from build123d import *

# Parameters (mm, degrees)
SKETCH_3_R          = 2
CUT_EXTRUDE_1_DEPTH = 10


with BuildPart() as part:
    # 草图1 → 旋转3 (revolve)
    with BuildSketch(Plane.XY):
        with BuildLine():
            Line((-14.38749457, 17), (-12.38749457, 17))
            Line((-12.38749457, 17), (-12.38749457, 6.523034438))
            ThreePointArc((-12.38749457, 6.523034438), (-13.590896291, 3.359693142), (-14, 0))
            Line((-14, 0), (-16, 0))
            ThreePointArc((-16, 0), (-15.591663047, 3.591663047), (-14.38749457, 7))
            Line((-14.38749457, 7), (-14.38749457, 17))
        make_face()
    revolve(axis=Axis((-26.155193714, 0, 0), (1, 0, 0)))

    # 草图2 → 切除-旋转1 (revolve, cut)
    with BuildSketch(Plane.XY):
        Polygon((-10.99354471, 5.03904502), (-18.623280316, 7.444691416), (-19.074339015, 6.01411599), (-11.444603409, 3.608469594), align=None)
    cut_revolve_1 = revolve(axis=Axis((0, 0, 0), (-0.9537169507482267, 0.30070579950427373, 0)), mode=Mode.SUBTRACT)

    # 镜向1: 切除-旋转1 across plane
    add(cut_revolve_1.mirror(Plane.ZX), mode=Mode.SUBTRACT)

    # 草图3 → 切除-拉伸1 (cut)
    with BuildSketch(Plane.ZY.offset(14.38749457)):
        with Locations((0, 12)):
            Circle(SKETCH_3_R)
        with Locations((10.392304845, -6)):
            Circle(SKETCH_3_R)
        with Locations((-10.392304845, -6)):
            Circle(SKETCH_3_R)
    extrude(amount=-CUT_EXTRUDE_1_DEPTH, mode=Mode.SUBTRACT)


solid = part.part
Build history of the part. All positions in model axes, mm. Round coordinates to 2 decimals unless told otherwise and drop trailing zeros. Loops run counter-clockwise (first coordinate to the right, second up) from the corner with the lowest first, then second, coordinate; pieces in that order, holes last. Notation, with made-up numbers: (-6, 15.5) -> (43, 15.5) arc R16 ccw to (43, 23.5) -> close; hole circle Ø7 at (59, 5.25). An arc over 180 degrees is marked (long way). Use CSV: the item, a comma, the result in double quotes. Start each with the question number.
Q1. Saw through at C-C on z = 0. Give the cut face in (x, y), and give its area (3 significant figures).
Q2. Saw through at B-B on z = -10.5. Give the cut face in (x, y).
Q3. Flat gauge pins, fed straight in: pin 1 Ø2 at (x, z) = (-13, -11) entering from -Y; pin 2 Ø5 at (y, z) = (-3, -1) entering from -X; pin 3 Ø12 at (y, z) = (8, -12) entering from -X. Where does each tip first touch, or does it go through?
Q4. Saw through at A-A on y = 0. Give the cut face in (x, z), and give its area (3 significant figures).
Q5. Drill centre lines: L1, parallel to X at y = 0, z = -10.5; L2, parallel to Y at x = -13.3, z = -1; L3, parallel to Y at x = -14.65, z = 1. Where is each one in solid material? Low to high.
Q6. Saw through at D-D on y = 12. Give the cut face in (x, z), and give its area (3 significant figures).
Q7. Mould opens along Z. For faces 1 (the face through (-13.373, 9.139, 14.334)), 2 (the face through (-14.387, 0.2, -7.3)), 3 (the face through (-13.401, -7.217, -11.979)) say: +Z half, -Z half, draft (parallel to the pull), parting line (faces both ways), or undercut.
Solutions:
1,outline,"(-15.64, -3.36) -> (-13.73, -2.76) arc R14 cw to (-13.73, 2.76) -> (-15.64, 3.36) arc R16 ccw to start; (-14.74, -6.22) arc R16 ccw to (-14.39, -7) -> (-14.39, -17) -> (-12.39, -17) -> (-12.39, -6.52) arc R14 cw to (-12.82, -5.62) -> close; (-14.74, 6.22) -> (-12.82, 5.62) arc R14 cw to (-12.39, 6.52) -> (-12.39, 10) -> (-14.39, 10) -> (-14.39, 7) arc R16 ccw to start; (-14.39, 14) -> (-12.39, 14) -> (-12.39, 17) -> (-14.39, 17) -> close"
1,area,"49.0 mm^2"
2,outline,"(-14.39, -13.37) -> (-12.39, -13.37) -> (-12.39, -8) -> (-14.39, -8) -> close; (-14.39, -4) -> (-12.39, -4) -> (-12.39, 13.37) -> (-14.39, 13.37) -> close"
3,pin 1,"stops at y = -13.75"
3,pin 2,"stops at x = -15.99"
3,pin 3,"stops at x = -14.39"
4,outline,"(-14.39, -17) -> (-12.39, -17) -> (-12.39, -6.52) arc R14 cw to (-12.39, 6.52) -> (-12.39, 17) -> (-14.39, 17) -> (-14.39, 7) arc R16 ccw to (-14.39, -7) -> close"
4,area,"69.0 mm^2"
5,L1,"x = -14.39 to -12.39"
5,L2,"y = -16.97 to -5.37, 5.37 to 10.27, 13.73 to 16.97"
5,L3,"y = -6.35 to -5.79, -3.45 to 3.45, 5.79 to 6.35"
6,outline,"(-14.39, -12.04) -> (-12.39, -12.04) -> (-12.39, -2) -> (-14.39, -2) -> close; (-14.39, 2) -> (-12.39, 2) -> (-12.39, 12.04) -> (-14.39, 12.04) -> close"
6,area,"40.2 mm^2"
7,face 1,"parting line"
7,face 2,"draft"
7,face 3,"undercut"
